from build123d import *

# Parameters (mm, degrees)
SKETCH1_R                  = 114.3
EXTRUDE1_DEPTH             = 6.35
SKETCH2_R                  = 93.6625
EXTRUDE2_DEPTH             = 15.875
SKETCH3_R                  = 87.3125
CUT_EXTRUDE1_DEPTH         = 15.875
SKETCH4_W                  = 3.175
SKETCH4_H                  = 2.54
CHAMFER1_SIZE              = 1.27
CHAMFER2_SIZE              = 0.635
SKETCH9_R                  = 6.35
CUT_EXTRUDE2_DEPTH         = 23.225
SKETCH11_R                 = 5.55625
CUT_EXTRUDE4_DEPTH         = 23.225
SKETCH12_R                 = 6.35
CUT_EXTRUDE5_DEPTH         = 23.225
SKETCH13_R                 = 5.55625
CUT_EXTRUDE6_DEPTH         = 23.225
SKETCH17_R                 = 92.3925
SKETCH17_R_2               = 69.85
BOSS_EXTRUDE1_DEPTH        = 5.08
F_12_24_TAPPED_HOLE1_D     = 4.4958
F_12_24_TAPPED_HOLE1_DEPTH = 14.224
F_8_32_TAPPED_HOLE1_D      = 3.4544
F_8_32_TAPPED_HOLE1_DEPTH  = 10.668
SKETCH25_R                 = 5.588
CUT_EXTRUDE8_DEPTH         = 28.305
SKETCH24_R                 = 6.35
CUT_EXTRUDE7_DEPTH         = 7.35
SKETCH26_R                 = 5.588
CUT_EXTRUDE9_DEPTH         = 28.305
SKETCH27_R                 = 5.55625
CUT_EXTRUDE10_DEPTH        = 28.305
SKETCH28_R                 = 6.062568313
CUT_EXTRUDE11_DEPTH        = 28.305


with BuildPart() as part:
    # Sketch1 → Extrude1 (new body)
    with BuildSketch(Plane.XY):
        Circle(SKETCH1_R)
    extrude(amount=EXTRUDE1_DEPTH)

    # Sketch2 → Extrude2 (add)
    with BuildSketch(Plane(origin=(0, 0, 0), x_dir=(-1, 0, 0), z_dir=(0, 0, -1))):
        Circle(SKETCH2_R)
    extrude(amount=EXTRUDE2_DEPTH)

    # Sketch3 → Cut-Extrude1 (cut)
    with BuildSketch(Plane(origin=(0, 0, -15.875), x_dir=(-1, 0, 0), z_dir=(0, 0, -1))):
        Circle(SKETCH3_R)
    extrude(amount=-CUT_EXTRUDE1_DEPTH, mode=Mode.SUBTRACT)

    # Sketch4 → Cut-Revolve1 (revolve, cut)
    with BuildSketch(Plane(origin=(0, 0, 0), x_dir=(0, 0, -1), z_dir=(1, 0, 0))):
        with Locations((4.395911794, 92.3925)):
            Rectangle(SKETCH4_W, SKETCH4_H)
        with Locations((10.251990741, 92.3925)):
            Rectangle(SKETCH4_W, SKETCH4_H)
    revolve(axis=Axis((0, 0, 0), (0, 0, -1)), mode=Mode.SUBTRACT)

    # Chamfer1
    chamfer1_edges = [part.edges().sort_by_distance(p)[0] for p in [
        (93.6625, 0, -15.875),
    ]]
    chamfer(chamfer1_edges, length=CHAMFER1_SIZE)

    # Chamfer2
    chamfer2_edges = [part.edges().sort_by_distance(p)[0] for p in [
        (93.6625, 0, -2.808411794),
        (93.6625, 0, -5.983411794),
        (93.6625, 0, -8.664490741),
        (93.6625, 0, -11.839490741),
    ]]
    chamfer(chamfer2_edges, length=CHAMFER2_SIZE)

    # Sketch9 → Cut-Extrude2 (cut, through all)
    with BuildSketch(Plane.XY.offset(6.35)):
        with Locations((-48.26, -38.1)):
            Circle(SKETCH9_R)
        with Locations((48.26, -38.1)):
            Circle(SKETCH9_R)
    extrude(amount=-CUT_EXTRUDE2_DEPTH, mode=Mode.SUBTRACT)

    # Sketch11 → Cut-Extrude4 (cut, through all)
    with BuildSketch(Plane.XY.offset(6.35)):
        with Locations((25.758421832, 62.186331333)):
            Circle(SKETCH11_R)
        with Locations((47.595357442, 47.595357442)):
            Circle(SKETCH11_R)
        with Locations((-47.595357442, 47.595357442)):
            Circle(SKETCH11_R)
        with Locations((-25.758421832, 62.186331333)):
            Circle(SKETCH11_R)
        with Locations((0, 67.31)):
            Circle(SKETCH11_R)
    extrude(amount=-CUT_EXTRUDE4_DEPTH, mode=Mode.SUBTRACT)

    # Sketch12 → Cut-Extrude5 (cut, through all)
    with BuildSketch(Plane.XY.offset(6.35)):
        with Locations((0, -57.15)):
            Circle(SKETCH12_R)
        with Locations((-25.4, 0)):
            Circle(SKETCH12_R)
        with Locations((25.4, 0)):
            Circle(SKETCH12_R)
    extrude(amount=-CUT_EXTRUDE5_DEPTH, mode=Mode.SUBTRACT)

    # Sketch13 → Cut-Extrude6 (cut, through all)
    with BuildSketch(Plane.XY.offset(6.35)):
        with Locations((0, 44.45)):
            Circle(SKETCH13_R)
        with Locations((28.571909251, 34.050675497)):
            Circle(SKETCH13_R)
        with Locations((-28.571909251, 34.050675497)):
            Circle(SKETCH13_R)
    extrude(amount=-CUT_EXTRUDE6_DEPTH, mode=Mode.SUBTRACT)

    # Sketch17 → Boss-Extrude1 (add)
    with BuildSketch(Plane(origin=(0, 0, -15.875), x_dir=(-1, 0, 0), z_dir=(0, 0, -1))):
        Circle(SKETCH17_R)
        Circle(SKETCH17_R_2, mode=Mode.SUBTRACT)
    extrude(amount=BOSS_EXTRUDE1_DEPTH)

    # #12-24 Tapped Hole1
    with Locations(Plane(origin=(0, 0, -20.955), x_dir=(-1, 0, 0), z_dir=(0, 0, -1))):
        with Locations((0, 79.375), (-79.375, 0), (0, -79.375), (79.375, 0)):
            Hole(F_12_24_TAPPED_HOLE1_D / 2, depth=F_12_24_TAPPED_HOLE1_DEPTH)

    # #8-32 Tapped Hole1
    with Locations(Plane.XY.offset(6.35)):
        with Locations((0, 101.6), (-86.20809861, -49.772268939), (87.988181024, -50.8)):
            Hole(F_8_32_TAPPED_HOLE1_D / 2, depth=F_8_32_TAPPED_HOLE1_DEPTH)

    # Sketch25 → Cut-Extrude8 (cut, through all)
    with BuildSketch(Plane.XY.offset(6.35)):
        with Locations((60.96, -10.16)):
            Circle(SKETCH25_R)
        with Locations((-60.96, -10.16)):
            Circle(SKETCH25_R)
    extrude(amount=-CUT_EXTRUDE8_DEPTH, mode=Mode.SUBTRACT)

    # Sketch24 → Cut-Extrude7 (cut, through all)
    with BuildSketch(Plane(origin=(0, 0, 0), x_dir=(-1, 0, 0), z_dir=(0, 0, -1))):
        with Locations((50.8, 25.4)):
            Circle(SKETCH24_R)
    extrude(amount=-CUT_EXTRUDE7_DEPTH, mode=Mode.SUBTRACT)

    # Sketch26 → Cut-Extrude9 (cut, through all)
    with BuildSketch(Plane.XY.offset(6.35)):
        with Locations((50.8, 25.4)):
            Circle(SKETCH26_R)
    extrude(amount=-CUT_EXTRUDE9_DEPTH, mode=Mode.SUBTRACT)

    # Sketch27 → Cut-Extrude10 (cut, through all)
    with BuildSketch(Plane.XY.offset(6.35)):
        with Locations((0, -24.13)):
            Circle(SKETCH27_R)
    extrude(amount=-CUT_EXTRUDE10_DEPTH, mode=Mode.SUBTRACT)

    # Sketch28 → Cut-Extrude11 (cut, through all)
    with BuildSketch(Plane.XY.offset(6.35)):
        with Locations((0, 23.787786302)):
            Circle(SKETCH28_R)
    extrude(amount=-CUT_EXTRUDE11_DEPTH, mode=Mode.SUBTRACT)


solid = part.part
Verification items for the finished model (mm, model axes). A direction names the side the tool comes from. Give positions to 0.01 mm unless a question says otherwise; leave off trailing zeros. Answer as a JSON object with one key per item and string values. Group by question number.
1) Cross-section at A-A (y = -38.1). Give the number of separate pieces and of enclosed holes in the cut face, then the cut area to 3 significant figures.
2) Mould release check, pull along Z, two halves, no side actions. Record for faces 1 (the face through (24.554, 56.762, 3.219)), 2 (the face through (-2, 2, 6.35)), 3 (the face through (-62, -68, -2.808)): released by +Z, released by -Z, zero draft, split by the parting line, or undercut.
3) Access from +Z, -Z, +X, -X, +Y, -Y to the whole of each face (thin tool, end or side, straight path). Record for faces 4 (the face through (18.928, -85.236, -8.049)), 5 (the face through (-0.72, 72.82, 3.22)), 6 (the face through (55.431, -42.503, -18.379)).
4) Depth check by flat-ended pin: pin 1 Ø2 at (x, z) = (48.5, -0.5) entering from +Y; pin 2 Ø6.5 at (x, y) = (-28.57, 34.05) entering from +Z; pin 3 Ø3 at (x, z) = (16, -16) entering from -Y; pin 4 Ø5 at (x, z) = (-39, -4) entering from -Y. Enter the tip coordinate at first touch or a pass-through.
5) Scan lines: line 1 along X through (y, z) = (-40.5, 3.75); line 2 along Z through (x, y) = (63, -78); line 3 along Z through (x, y) = (79, 2.5) (3 decimals). Record each from-to range of solid material in increasing order. Write a range as [from, to].
Result sheet:
{
 "1": {"separate pieces": "3", "enclosed holes": "0", "area": "1,650 mm2"},
 "2": {"face 1": "zero draft", "face 2": "released by +Z", "face 3": "undercut"},
 "3": {"face 4": "none", "face 5": "+Z", "face 6": "-Z"},
 "4": {"pin 1": "stops at y = 103.9", "pin 2": "passes through", "pin 3": "stops at y = -92.38", "pin 4": "stops at y = -85.92"},
 "5": {"line 1": "x = [-106.88, -54.14], [-42.38, 42.38], [54.14, 106.88]", "line 2": "z = [0, 6.35]", "line 3": "z = [-20.955, -15.875], [0, 6.35]"}
}
